Geometry: final body of the model. Coordinates: model frame, mm. Coordinates: 2 decimals unless noted, no trailing zeros. Write each loop counter-clockwise with the first axis right and the second up, starting at its lowest first coordinate (ties: lowest second). Pieces come first, ordered by that corner, then holes. Notation, with made-up numbers: (61, 63) -> (105, 63) arc R34 cw to (105, 99) -> close; hole circle Ø2 at (23, -35.75). An arc over 180 degrees is marked (long way). One line per item, written item: value.
```python
from build123d import *

# Parameters (mm, degrees)
F0_W     = 1590.675
F0_H     = 101.6
F1_DEPTH = 16
F2_W     = 410.9626214183
F2_H     = 50.8
F2_W_2   = 419.1
F3_DEPTH = 25.4


with BuildPart() as f1:
    # F0 (on Front) → F1 (new body)
    with BuildSketch(Plane.XZ):
        with Locations((18.1653643548, -22.8088884252)):
            Rectangle(F0_W, F0_H)
    extrude(amount=F1_DEPTH)

    # F2 (on face) → F3 (cut)
    with BuildSketch(Plane.XZ.offset(16)):
        with BuildLine():
            Line((-642.0347570634, -73.6088884252), (-642.0347570634, -22.8088884252))
            ThreePointArc((-642.0347570634, -22.8088884252), (-685.9453309895, -36.797837184), (-713.6721356452, -73.6088884252))
            Line((-713.6721356452, -73.6088884252), (-642.0347570634, -73.6088884252))
        make_face()
        with Locations((-436.5534463543, -48.2088884252)):
            Rectangle(F2_W, F2_H)
        with BuildLine():
            Line((-231.0721356452, -73.6088884252), (-167.5721356452, -73.6088884252))
            ThreePointArc((-167.5721356452, -73.6088884252), (-190.4122967375, -37.0715897906), (-231.0721356452, -22.8088884252))
            Line((-231.0721356452, -22.8088884252), (-231.0721356452, -73.6088884252))
        make_face()
        with BuildLine():
            ThreePointArc((267.4028643548, -22.8088884252), (226.7430254472, -37.0715897906), (203.9028643548, -73.6088884252))
            Line((203.9028643548, -73.6088884252), (267.4028643548, -73.6088884252))
            Line((267.4028643548, -73.6088884252), (267.4028643548, -22.8088884252))
        make_face()
        with Locations((476.9528643548, -48.2088884252)):
            Rectangle(F2_W_2, F2_H)
        with BuildLine():
            ThreePointArc((750.0028643548, -73.6088884252), (727.1627032625, -37.0715897906), (686.5028643548, -22.8088884252))
            Line((686.5028643548, -22.8088884252), (686.5028643548, -73.6088884252))
            Line((686.5028643548, -73.6088884252), (750.0028643548, -73.6088884252))
        make_face()
    extrude(amount=-F3_DEPTH, mode=Mode.SUBTRACT)


solid = f1.part
```
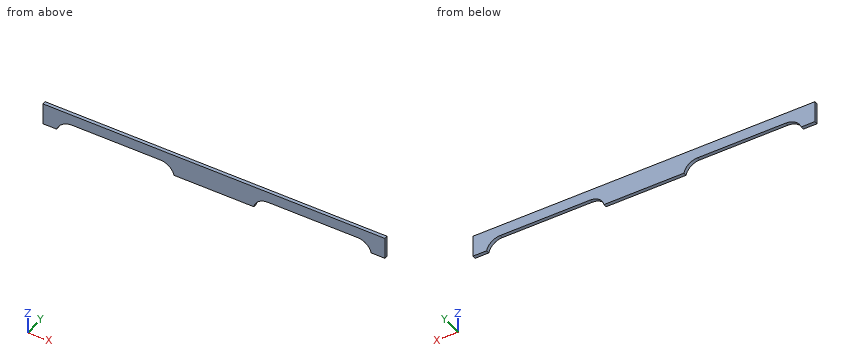
(1) First-contact query: pin 1 (5 mm diameter, centred on x = 515.5, y = -9, fed in from -Z). Flat tip, straight axial feed; report the tip coordinate or a pass-through.
Responses:
pin 1: stops at z = -22.81
(2) Section C-C (x = -348). Return the cut outline in (y, z).
Responses:
outline: (-16, -22.81) -> (0, -22.81) -> (0, 27.99) -> (-16, 27.99) -> close
(3) Section A-A (z = -47.5). Return the cut outline in (x, y), then the cut area to 3 significant figures.
Responses:
outline: (-777.17, -16) -> (-698.06, -16) -> (-698.06, 0) -> (-777.17, 0) -> close; (-180.04, -16) -> (216.37, -16) -> (216.37, 0) -> (-180.04, 0) -> close; (737.54, -16) -> (813.5, -16) -> (813.5, 0) -> (737.54, 0) -> close
area: 8,820 mm2
(4) Line query: line 1 (X direction, y = -2.75, z = -43); line 2 (X direction, y = -10, z = -61.5); line 3 (Z direction, x = -449.5, y = -1.5). Output: solid intervals per line, ascending. Write a range as [from, to].
Responses:
line 1: x = [-777.17, -693.59], [-183.95, 220.28], [733.63, 813.5]
line 2: x = [-777.17, -708.19], [-171.58, 207.91], [746, 813.5]
line 3: z = [-22.81, 27.99]
(5) Section D-D (x = 227). Return the cut outline in (y, z).
Responses:
outline: (-16, -36.87) -> (0, -36.87) -> (0, 27.99) -> (-16, 27.99) -> close
(6) Section B-B (y = -8.5). Return the cut outline in (x, z) (1 decimal), then the cut area to 3 significant figures.
Responses:
outline: (-777.2, -73.6) -> (-713.7, -73.6) arc R75.9 cw to (-642, -22.8) -> (-231.1, -22.8) arc R65.1 cw to (-167.6, -73.6) -> (203.9, -73.6) arc R65.1 cw to (267.4, -22.8) -> (686.5, -22.8) arc R65.1 cw to (750, -73.6) -> (813.5, -73.6) -> (813.5, 28) -> (-777.2, 28) -> close
area: 110,000 mm2
